```python
from build123d import *

# Parameters (mm, degrees)
F1_DEPTH = 7.62
F2_R     = 11.0625
F3_DEPTH = 10
F4_R     = 3


with BuildPart() as f1:
    # F0 (on Front) → F1 (new body)
    with BuildSketch(Plane.XZ):
        Polygon((0, 2.178027), (-6.844124, 6.442403), (-16.118215, 6.442403), (-25.278939, 0), (-36.931682, 0), (-33.736575, -13.062352), (-26.406623, -22.271778), (-13.536484, -31.557597), (0, -29.661065), (14.002089, -32.608893), (23.587411, -27.53431), (34.112468, -15.129773), (38.62321, 0), (25.466887, 0), (14.694345, 6.442403), (6.435679, 6.442403), align=None)
    extrude(amount=F1_DEPTH)

    # F2 (on face) → F3 (cut)
    with BuildSketch(Plane.XZ.offset(7.62)):
        with Locations((0, -13.812818)):
            Circle(F2_R)
    extrude(amount=-F3_DEPTH, mode=Mode.SUBTRACT)

    # F4
    f4_edges = [f1.edges().sort_by_distance(p)[0] for p in [
        (-35.334129, -7.62, -6.531176),
        (-30.071599, -7.62, -17.667065),
        (-19.971554, -7.62, -26.914688),
        (-6.768242, -7.62, -30.609331),
        (7.001045, -7.62, -31.134979),
        (18.79475, -7.62, -30.071601),
        (28.84994, -7.62, -21.332041),
        (36.367839, -7.62, -7.564886),
        (32.045049, -7.62, 0),
        (20.080616, -7.62, 3.221201),
        (10.565012, -7.62, 6.442403),
        (3.21784, -7.62, 4.310215),
        (-3.422062, -7.62, 4.310215),
        (-11.481169, -7.62, 6.442403),
        (-20.698577, -7.62, 3.221201),
        (-31.105311, -7.62, 0),
        (-31.105311, 0, 0),
        (-35.334129, 0, -6.531176),
        (-30.071599, 0, -17.667065),
        (-19.971554, 0, -26.914688),
        (-6.768242, 0, -30.609331),
        (7.001045, 0, -31.134979),
        (18.79475, 0, -30.071601),
        (28.84994, 0, -21.332041),
        (36.367839, 0, -7.564886),
        (32.045049, 0, 0),
        (20.080616, 0, 3.221201),
        (10.565012, 0, 6.442403),
        (3.21784, 0, 4.310215),
        (-3.422062, 0, 4.310215),
        (-11.481169, 0, 6.442403),
        (-20.698577, 0, 3.221201),
    ]]
    fillet(f4_edges, radius=F4_R)


solid = f1.part
```
Input: part model. Units: mm. Frame: model coordinates. A direction names the side the tool comes from. Give positions to 0.01 mm unless a question says otherwise; leave off trailing zeros. Order: outer loops, then holes, each group sorted by start corner. A loop starts at its lowest first (then second) coordinate and runs counter-clockwise, first axis right, second up. Notation, with made-up numbers: (18.5, 42.25) - (31.5, 42.25) arc R15 ccw to (31.5, 50.25) - close; hole circle Ø8 at (19, -13.75). An arc over 180 degrees is marked (long way). Use a Markdown table: item, result.
(1) Line query: line 1 (X direction, y = -5, z = -14.5); line 2 (Z direction, x = -3.5, y = -6.25); line 3 (X direction, y = -3.25, z = -19). Output: solid intervals per line, ascending. Write a range as from..to.
Computed values:
| item | result |
|---|---|
| line 1 | x = -32.56..-11.04, 11.04..34.28 |
| line 2 | z = -29.67..-24.31, -3.32..3.79 |
| line 3 | x = -29.01..-9.77, 9.77..30.83 |
(2) Section query A-A (y = -0.75). Output: boundary loops of the cut face in (x, z) (1 decimal).
Computed values:
| item | result |
|---|---|
| outline | (-35.6, -1) - (-32.8, -12.6) - (-25.7, -21.5) - (-13.3, -30.5) - (0, -28.6) - (13.9, -31.5) - (22.9, -26.7) - (33.2, -14.6) - (37.3, -1) - (25.2, -1) - (14.4, 5.4) - (6.7, 5.4) - (0, 1) - (-7.1, 5.4) - (-15.8, 5.4) - (-25, -1) - close; hole circle Ø22.1 at (0, -13.8) |
(3) Pin query (flat end, axial travel): pin 1 (3 mm diameter, centred on x = 10, y = -1, fed in from -Z); pin 2 (1.5 mm diameter, centred on y = -2.5, z = -25, fed in from +X); pin 3 (1.8 mm diameter, centred on x = -31.5, y = -3.5, fed in from +Z). Return the tip coordinate at first contact, or that it passes through.
Computed values:
| item | result |
|---|---|
| pin 1 | stops at z = -31.84 |
| pin 2 | stops at x = 26.33 |
| pin 3 | stops at z = 0 |
(4) Draft query along X for faces 1 (the flat face through (3.26, -3.8, 4.34)), 2 (the flat face through (-31, -4, 0)), 3 (the cylindrical face through (-29.314, -6.765, -17.17)). Return one class per face: released by +X, released by -X, zero draft, split by the parting line, or undercut.
Computed values:
| item | result |
|---|---|
| face 1 | undercut |
| face 2 | zero draft |
| face 3 | released by -X |
(5) Access query for faces 4 (the flat face through (-3.37, -3.8, 4.28)), 5 (the cylindrical face through (-30.72, -0.86, -0.9)), 6 (the flat face through (6.903, -3.799, -31.114)), 7 (the cylindrical face through (-3.1, -0.9, 3.1)). Directions: +Z, -Z, +X, -X, +Y, -Y. A direction counts if a zero-diameter tool reaches every point of the face in a straight line with its end or side. Return the directions, or none.
Computed values:
| item | result |
|---|---|
| face 4 | +Z, +Y, -Y |
| face 5 | +Z, -X, +Y |
| face 6 | -Z, +Y, -Y |
| face 7 | +Z, +Y |
